Design review of the part built by this model. Coordinates are the model's own, in mm. Face numbers are marked on the shaded views. A direction names the side the tool comes from. Coordinates: 2 decimals unless noted, no trailing zeros. Loops run counter-clockwise (first coordinate to the right, second up) from the corner with the lowest first, then second, coordinate; pieces in that order, holes last. Notation, with made-up numbers: M 29.25,7 L 40.25,7 A20 ccw 40.25,42 Z; hole C -32,-39 d2. An arc over 180 degrees is marked long. Put each result on its own line as item: value. Start each with the question number.
(1) Clearance check with flat-ended pins moving along their axes: pin 1 (9.5 mm diameter, centred on x = 53.5, y = 0, fed in from -Z); pin 2 (2 mm diameter, centred on x = -7, y = 4.5, fed in from -Z); pin 3 (3 mm diameter, centred on x = -10.5, y = 0, fed in from +Z); pin 4 (2 mm diameter, centred on x = 13, z = 3.5, fed in from -Y). State where each tip first meets the part, or that it passes through.
(2) The part is to be moulded in two halves that separate along X. For the marked faces 4, 5 and 6, say which applies: +X half, -X half, draft (parallel to the pull), parting line (faces both ways), or undercut.
(3) Take a section at C-C, the plane z = 3.75. Give the boundary of the cut face in (x, y), then the cut area to 3 significant figures.
(4) Take a section at D-D, the plane x = 25. Give the boundary of the cut face in (y, z).
(5) For the marked faces 1, 2 and 3, list the 3-axis set-ups (+Z, -Z, +X, -X, +Y, -Y) from which the entire face can be reached by the end or side of a thin tool; tool diameter is ignored.
(6) Take a section at B-B, the plane x = 53.5. Give the boundary of the cut face in (y, z).
(7) For probe 1 along Y at (x, z) = (3, 1.5); probe 2 along Z at (x, y) = (-24, -9); probe 3 along Y at (x, z) = (53.5, 0.8), list the stretches that pass through material, from the lowest coordinate up. Write a range as [from, to].
(8) Take a section at A-A, the plane y = 0. Give the boundary of the cut face in (x, z).
```python
from build123d import *

# Parameters (mm, degrees)
PAD009_DEPTH    = 8
THICKNESS_T     = -1.4
SKETCH017_R     = 7.75
POCKET006_DEPTH = 1.401


with BuildPart() as part:
    # Sketch016 → Pad009 (new body)
    with BuildSketch(Plane.XY):
        with BuildLine():
            Line((-8.657434, 10.75), (64, 10.75))
            Line((64, 10.75), (64, -10.75))
            Line((64, -10.75), (-8.657434, -10.75))
            Line((-19.999998, -12.75), (-8.657434, -10.75))
            ThreePointArc((-19.999998, 12.75), (-32.75, 0), (-19.999998, -12.75))
            Line((-19.999998, 12.75), (-8.657434, 10.75))
        make_face()
    extrude(amount=PAD009_DEPTH)

    # Thickness
    thickness_openings = [part.faces().sort_by_distance(p)[0] for p in [
        (15.774779, 0, 8),
    ]]
    offset(amount=THICKNESS_T, openings=thickness_openings)

    # Sketch017 (on Face17 of Thickness) → Pocket006 (cut, through all)
    with BuildSketch(Plane.XY.offset(1.4)):
        with Locations((53.5, 0)):
            Circle(SKETCH017_R)
    extrude(amount=-POCKET006_DEPTH, mode=Mode.SUBTRACT)


solid = part.part
```
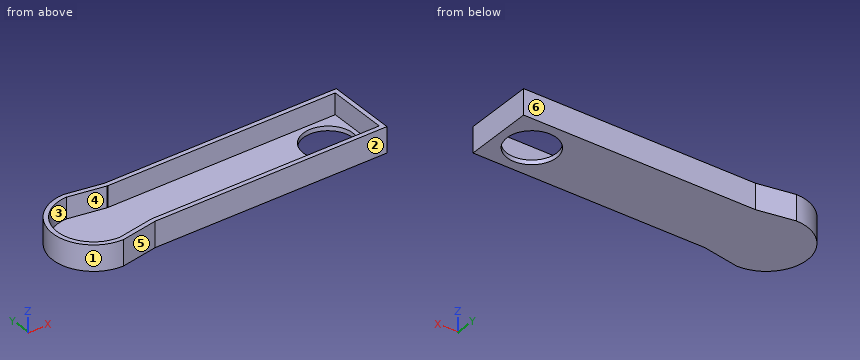
Computed values:
1. pin 1: passes through
1. pin 2: stops at z = 0
1. pin 3: stops at z = 1.4
1. pin 4: stops at y = -10.75
2. face 4: undercut
2. face 5: +X half
2. face 6: draft
3. outline: M -20,-12.75 L -8.66,-10.75 L 64,-10.75 L 64,10.75 L -8.66,10.75 L -20,12.75 A12.75 ccw Z; hole M -20.12,-11.35 L -8.9,-9.37 A1.4 cw -8.66,-9.35 L 62.6,-9.35 L 62.6,9.35 L -8.66,9.35 A1.4 cw -8.9,9.37 L -20.12,11.35 A11.35 ccw Z
3. area: 315 mm^2
4. outline: M -10.75,0 L 10.75,0 L 10.75,8 L 9.35,8 L 9.35,1.4 L -9.35,1.4 L -9.35,8 L -10.75,8 Z
5. face 1: +Z, -Z, -X
5. face 2: +Z, -Z, +X, -Y
5. face 3: +Z
6. outline: M -10.75,0 L -7.75,0 L -7.75,1.4 L -9.35,1.4 L -9.35,8 L -10.75,8 Z; M 7.75,0 L 10.75,0 L 10.75,8 L 9.35,8 L 9.35,1.4 L 7.75,1.4 Z
7. probe 1: y = [-10.75, -9.35], [9.35, 10.75]
7. probe 2: z = [0, 1.4]
7. probe 3: y = [-10.75, -7.75], [7.75, 10.75]
8. outline: M -32.75,0 L 45.75,0 L 45.75,1.4 L -31.35,1.4 L -31.35,8 L -32.75,8 Z; M 61.25,0 L 64,0 L 64,8 L 62.6,8 L 62.6,1.4 L 61.25,1.4 Z
